from build123d import *

# Parameters (mm, degrees)
BOSS_EXTRUDE2_DEPTH     = 2
FILLET1_R               = 2
FILLET2_R               = 10
ECHELLE1_SCALE          = 2
ESQUISSE1_W             = 16
ESQUISSE1_H             = 4.343145751
BOSS_EXTRU_1_DEPTH      = 23
ENL_V_MAT_EXTRU_1_REACH = 108.536
ESQUISSE2_R             = 1.7
CONG_1_R                = 5


with BuildPart() as part:
    # Sketch2 → Boss-Extrude2 (new body)
    with BuildSketch(Plane(origin=(0, 0, 0), x_dir=(1, 0, 0), z_dir=(0, 1, 0))):
        Polygon((4, 6), (32.284271247, 34.284271247), (35.819805153, 30.748737342), (10, 4.928932188), (10, -4.928932188), (35.819805153, -30.748737342), (32.284271247, -34.284271247), (4, -6), (4, -3), (-4, -3), (-4, -6), (-32.284271247, -34.284271247), (-35.819805153, -30.748737342), (-10, -4.928932188), (-10, 4.928932188), (-35.819805153, 30.748737342), (-32.284271247, 34.284271247), (-4, 6), (-4, 3), (4, 3), align=None)
    extrude(amount=BOSS_EXTRUDE2_DEPTH)

    # Fillet1
    fillet1_edges = [part.edges().sort_by_distance(p)[0] for p in [
        (4, 1, -6),
        (32.284271247, 1, -34.284271247),
        (35.819805153, 1, -30.748737342),
        (35.819805153, 1, 30.748737342),
        (32.284271247, 1, 34.284271247),
        (4, 1, 6),
        (-4, 1, 6),
        (-32.284271247, 1, 34.284271247),
        (-35.819805153, 1, 30.748737342),
        (-35.819805153, 1, -30.748737342),
        (-32.284271247, 1, -34.284271247),
        (-4, 1, -6),
    ]]
    fillet(fillet1_edges, radius=FILLET1_R)

    # Fillet2
    fillet2_edges = [part.edges().sort_by_distance(p)[0] for p in [
        (10, 1, -4.928932188),
        (10, 1, 4.928932188),
        (-10, 1, 4.928932188),
        (-10, 1, -4.928932188),
    ]]
    fillet(fillet2_edges, radius=FILLET2_R)


with BuildPart() as part_1:
    # Echelle1: scaled about (0, 1, 0)
    add(part.part.scale(ECHELLE1_SCALE).moved(Location((0, -1, 0))))

    # Esquisse1 → Boss.-Extru.1 (add)
    with BuildSketch(Plane.XZ.offset(1)):
        with Locations((0, -8.171572876)):
            Rectangle(ESQUISSE1_W, ESQUISSE1_H)
        with Locations((0, 8.171572876)):
            Rectangle(ESQUISSE1_W, ESQUISSE1_H)
    extrude(amount=-BOSS_EXTRU_1_DEPTH)

    # Enlèv. mat.-Extru.1: up to this face of the body (flat: up to its plane)
    enl_v_mat_extru_1_end = Plane(part_1.part.faces().sort_by_distance((0, 10.5, 10.343145751))[0])
    # Esquisse2 → Enlèv. mat.-Extru.1 (cut, up to the picked face)
    with BuildSketch(Plane(origin=(0, 0, -10.343145751), x_dir=(-1, 0, 0), z_dir=(0, 0, -1)), mode=Mode.PRIVATE) as enl_v_mat_extru_1_sk1:
        with Locations((0, 17.955923501)):
            Circle(ESQUISSE2_R)
    enl_v_mat_extru_1_tool1 = split(extrude(enl_v_mat_extru_1_sk1.sketch, amount=-ENL_V_MAT_EXTRU_1_REACH, mode=Mode.PRIVATE), bisect_by=enl_v_mat_extru_1_end, keep=Keep.BOTH, mode=Mode.PRIVATE)
    add(enl_v_mat_extru_1_tool1.solids().sort_by(Axis((0, 17.955924, -10.343146), (0, 0, 1)))[0], mode=Mode.SUBTRACT)

    # Congé1
    cong_1_edges = [part_1.edges().sort_by_distance(p)[0] for p in [
        (8, 22, -8.171572875),
        (-8, 22, -8.171572875),
        (8, 22, 8.171572875),
        (-8, 22, 8.171572875),
    ]]
    fillet(cong_1_edges, radius=CONG_1_R)


solid = part_1.part
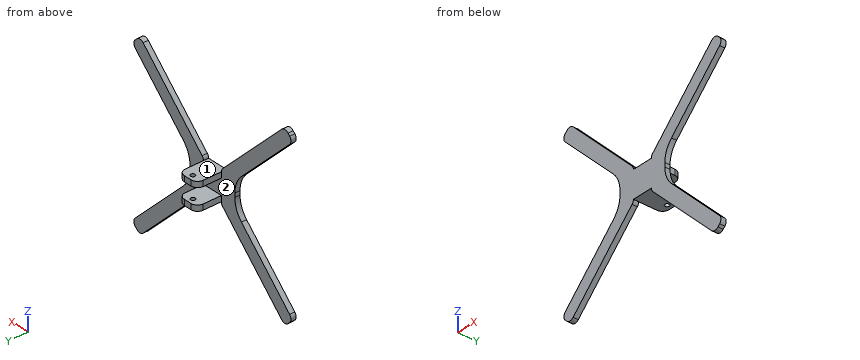
Here's how the part is built. I have some questions about the finished solid (model axes, mm). Face numbers are marked on the shaded views. Give positions to 0.01 mm unless a question says otherwise; leave off trailing zeros. Order: outer loops, then holes, each group sorted by start corner. A loop starts at its lowest first (then second) coordinate and runs counter-clockwise, first axis right, second up. Notation, with made-up numbers: M 13.25,1.25 L 55.25,1.25 A13 ccw 55.25,9.25 Z; hole C -18,-29 d2. An arc over 180 degrees is marked long. Answer as a JSON object with one key per item and string values. Group by question number.
1) Please list where these lines run through material, in increasing order: L1, parallel to Y at x = 0, z = -8; L2, parallel to Z at x = 1.5, y = 20.25; L3, parallel to Z at x = 32, y = 2.5. Write a range as [from, to].
2) Suppose I cut it at C-C, the plane z = 34. Write out the boundary of the cut face in (x, y), plus the area to 3 significant figures.
3) We'd pull the mould along X, two halves only. Please class the marked faces 1 and 2: pulls with the +X half, pulls with the -X half, needs draft (parallel to the pull), parting line crosses it, or undercut.
4) I'm going to push flat-ended pins straight in: pin 1 Ø2 at (y, z) = (7, 8.5) entering from -X; pin 2 Ø8 at (x, z) = (-15, 19) entering from +Y; pin 3 Ø8 at (x, y) = (3.5, 12) entering from -Z. Where does each tip first touch, or does it pass through?
5) Suppose I cut it at D-D, the plane z = -8.5. Write out the boundary of the cut face in (x, y), plus the area to 3 significant figures.
6) Suppose I cut it at A-A, the plane y = 12.75. Write out the boundary of the cut face in (x, z), plus the area to 3 significant figures.
7) Suppose I cut it at B-B, the plane x = 0. Write out the boundary of the cut face in (y, z).
Results found:
{
 "1": {"L1": "[-1, 16.26], [19.66, 22]", "L2": "[-10.34, -6], [6, 10.34]", "L3": "[-36, -21.86], [21.86, 36]"},
 "2": {"outline": "M -44.14,-1 L -30,-1 L -30,3 L -44.14,3 Z; M 30,-1 L 44.14,-1 L 44.14,3 L 30,3 Z", "area": "113 mm²"},
 "3": {"face 1": "undercut", "face 2": "needs draft"},
 "4": {"pin 1": "x = -8", "pin 2": "y = 3", "pin 3": "z = -10.34"},
 "5": {"outline": "M -21.24,-1 L 21.24,-1 L 21.24,3 L 8,3 L 8,17 A5 ccw 3,22 L -3,22 A5 ccw -8,17 L -8,3 L -21.24,3 Z; hole C 0,17.96 d3.4", "area": "454 mm²"},
 "6": {"outline": "M -8,-10.34 L 8,-10.34 L 8,-6 L -8,-6 Z; M -8,6 L 8,6 L 8,10.34 L -8,10.34 Z", "area": "139 mm²"},
 "7": {"outline": "M -1,-10.34 L 16.26,-10.34 L 16.26,-6 L 3,-6 L 3,6 L 16.26,6 L 16.26,10.34 L -1,10.34 Z; M 19.66,-10.34 L 22,-10.34 L 22,-6 L 19.66,-6 Z; M 19.66,6 L 22,6 L 22,10.34 L 19.66,10.34 Z"}
}
